Verification items for the finished model (mm, model axes). A direction names the side the tool comes from. Give positions to 0.01 mm unless a question says otherwise; leave off trailing zeros. Order: outer loops, then holes, each group sorted by start corner. A loop starts at its lowest first (then second) coordinate and runs counter-clockwise, first axis right, second up. Notation, with made-up numbers: (67.25, 85.5) -> (121.25, 85.5) arc R27 ccw to (121.25, 118.5) -> close; hole circle Ø9 at (74, 73.25). An arc over 180 degrees is marked (long way). One line per question, with ' | ' between items. Start each with the question number.
Q1. Section check D-D on z = 4.8. Record the cut outline in (x, y), plus the area to 3 significant figures.
Q2. Access from +Z, -Z, +X, -X, +Y, -Y to the whole of each face (thin tool, end or side, straight path). Record for faces 1 (the flat face through (-5.1, 2, 7)), 2 (the cylindrical face through (1.5, 2, -4.3)), 3 (the flat face through (-7, 2, 5)).
Q3. Section check A-A on z = 7.75. Record the cut outline in (x, y).
Q4. Mould release check, pull along X, two halves, no side actions. Record for faces 4 (the flat face through (7, 2, 5)), 5 (the cylindrical face through (-6.5, 2, 12.6)), 6 (the flat face through (-1, 0, 5)), 7 (the flat face through (-2.2, 2, -3)): released by +X, released by -X, zero draft, split by the parting line, or undercut.
Q5. Go/stop test with flat-tipped pins: pin 1 (0.6 mm diameter, centred on y = 1.5, z = -2.5, fed in from -X); pin 2 (0.6 mm diameter, centred on y = 1.5, z = -3.5, fed in from -X); pin 3 (1.9 mm diameter, centred on x = -4.5, y = 1, fed in from +Z). Record where each tip stops, or that it passes through.
Q6. Material ranges on probe 1 along X at (y, z) = (3.3, 2.75); probe 2 along X at (y, z) = (2.9, 4.75); probe 3 along X at (y, z) = (0.85, 5.25), recorded low to high. Write a range as [from, to].
Q7. Section check B-B on x = 0. Record the cut outline in (y, z).
Q8. Section check C-C on y = 3.5. Record the cut outline in (x, z).
from build123d import *

# Parameters (mm, degrees)
EXTRUDE_1_DEPTH     = 4
SKETCH_2_W          = 1.7
SKETCH_2_H          = 55.892000818
CUT_EXTRUDE_1_DEPTH = 19.814887722
CUT_EXTRUDE_2_DEPTH = 19.814887722
SKETCH_4_R          = 0.6
CUT_EXTRUDE_3_DEPTH = 19.814887722


with BuildPart() as part:
    # 草图1 → 凸台-拉伸1 (new body)
    with BuildSketch(Plane(origin=(0, 0, 0), x_dir=(1, 0, 0), z_dir=(0, 1, 0))):
        with BuildLine():
            Line((7, 0), (7, -10))
            ThreePointArc((7, -10), (0, -17), (-7, -10))
            Line((-7, -10), (-7, 0))
            ThreePointArc((-7, 0), (0, 7), (7, 0))
        make_face()
    extrude(amount=EXTRUDE_1_DEPTH)

    # 草图2 → 切除-拉伸1 (cut, through all)
    with BuildSketch(Plane(origin=(0, 4, 0), x_dir=(1, 0, 0), z_dir=(0, 1, 0))):
        with Locations((-4.25, -27.746000409)):
            Rectangle(SKETCH_2_W, SKETCH_2_H)
        with Locations((4.25, -27.746000409)):
            Rectangle(SKETCH_2_W, SKETCH_2_H)
    extrude(amount=-CUT_EXTRUDE_1_DEPTH, mode=Mode.SUBTRACT)

    # 草图3 → 切除-拉伸2 (cut, through all)
    with BuildSketch(Plane(origin=(0, 4, 0), x_dir=(1, 0, 0), z_dir=(0, 1, 0))):
        with BuildLine():
            Line((-2.2, 2.4), (-2.2, 3.6))
            ThreePointArc((-2.2, 3.6), (-1.5, 4.3), (-0.8, 3.6))
            Line((-0.8, 3.6), (-0.8, 2.4))
            ThreePointArc((-0.8, 2.4), (-1.5, 1.7), (-2.2, 2.4))
        make_face()
        with BuildLine():
            Line((2.2, 2.4), (2.2, 3.6))
            ThreePointArc((2.2, 3.6), (1.5, 4.3), (0.8, 3.6))
            Line((0.8, 3.6), (0.8, 2.4))
            ThreePointArc((0.8, 2.4), (1.5, 1.7), (2.2, 2.4))
        make_face()
    extrude(amount=-CUT_EXTRUDE_2_DEPTH, mode=Mode.SUBTRACT)

    # 草图4 → 切除-拉伸3 (cut, through all)
    with BuildSketch(Plane(origin=(0, 4, 0), x_dir=(1, 0, 0), z_dir=(0, 1, 0))):
        with Locations(Location((0, -4.8, 0), (0, 0, 270))):
            Circle(SKETCH_4_R)
    extrude(amount=-CUT_EXTRUDE_3_DEPTH, mode=Mode.SUBTRACT)


solid = part.part
Filled in:
1) outline: (-7, 0) -> (-5.1, 0) -> (-5.1, 4) -> (-7, 4) -> close; (-3.4, 0) -> (-0.6, 0) -> (-0.6, 4) -> (-3.4, 4) -> close; (0.6, 0) -> (3.4, 0) -> (3.4, 4) -> (0.6, 4) -> close; (5.1, 0) -> (7, 0) -> (7, 4) -> (5.1, 4) -> close | area: 37.6 mm²
2) face 1: +Z, +Y, -Y | face 2: +Y, -Y | face 3: +Z, -Z, -X, +Y, -Y
3) outline: (-7, 0) -> (-5.1, 0) -> (-5.1, 4) -> (-7, 4) -> close; (-3.4, 0) -> (3.4, 0) -> (3.4, 4) -> (-3.4, 4) -> close; (5.1, 0) -> (7, 0) -> (7, 4) -> (5.1, 4) -> close
4) face 4: released by +X | face 5: released by -X | face 6: zero draft | face 7: undercut
5) pin 1: x = -6.65 | pin 2: x = -6.23 | pin 3: z = 14.79
6) probe 1: [-7, -5.1], [-3.4, 3.4], [5.1, 7] | probe 2: [-7, -5.1], [-3.4, -0.6], [0.6, 3.4], [5.1, 7] | probe 3: [-7, -5.1], [-3.4, -0.4], [0.4, 3.4], [5.1, 7]
7) outline: (0, -7) -> (4, -7) -> (4, 4.2) -> (0, 4.2) -> close; (0, 5.4) -> (4, 5.4) -> (4, 17) -> (0, 17) -> close
8) outline: (-7, 0) arc R7 ccw to (7, 0) -> (7, 10) arc R7 ccw to (5.1, 14.79) -> (5.1, -0.2) -> (3.4, -0.2) -> (3.4, 16.12) arc R7 ccw to (-3.4, 16.12) -> (-3.4, -0.2) -> (-5.1, -0.2) -> (-5.1, 14.79) arc R7 ccw to (-7, 10) -> close; hole (-2.2, -3.6) arc R0.7 ccw to (-0.8, -3.6) -> (-0.8, -2.4) arc R0.7 ccw to (-2.2, -2.4) -> close; hole circle Ø1.2 at (0, 4.8); hole (0.8, -3.6) arc R0.7 ccw to (2.2, -3.6) -> (2.2, -2.4) arc R0.7 ccw to (0.8, -2.4) -> close
